Geometry: final body of the model. Coordinates: model frame, mm. Face numbers are marked on the shaded views. A direction names the side the tool comes from. Give positions to 0.01 mm unless a question says otherwise; leave off trailing zeros. Loops run counter-clockwise (first coordinate to the right, second up) from the corner with the lowest first, then second, coordinate; pieces in that order, holes last.
from build123d import *

# Parameters (mm, degrees)
PROFILESKETCH3_R               = 2.5
PROFILESKETCH3_R_2             = 2.3
PROFILEBOSS_EXTRUDE1_DEPTH     = 5.5
FILLET1_R                      = 1.5
SKETCH1_W                      = 20
SKETCH1_H                      = 15.75
SLIDINGMOUNTCUT_EXTRUDE1_DEPTH = 1


with BuildPart() as part:
    # ProfileSketch3 → ProfileBoss-Extrude1 (new body)
    with BuildSketch(Plane.XY):
        Polygon((0, 46.85), (15, 46.85), (15, 64.85), (0, 64.85), (0, 76.85), (20, 76.85), (20, 0), (0, 0), align=None)
        with Locations((7.5, 40.35)):
            Circle(PROFILESKETCH3_R, mode=Mode.SUBTRACT)
        with Locations((7.5, 71.35)):
            Circle(PROFILESKETCH3_R, mode=Mode.SUBTRACT)
        with Locations((15, 9.375)):
            Circle(PROFILESKETCH3_R_2, mode=Mode.SUBTRACT)
    extrude(amount=PROFILEBOSS_EXTRUDE1_DEPTH)

    # Fillet1
    fillet1_edges = [part.edges().sort_by_distance(p)[0] for p in [
        (7.5, 46.85, 0),
        (7.5, 64.85, 0),
    ]]
    fillet(fillet1_edges, radius=FILLET1_R)

    # Sketch1 → SlidingMountCut-Extrude1 (cut)
    with BuildSketch(Plane.XY.offset(5.5)):
        with Locations((10, 9.375)):
            Rectangle(SKETCH1_W, SKETCH1_H)
    extrude(amount=-SLIDINGMOUNTCUT_EXTRUDE1_DEPTH, mode=Mode.SUBTRACT)


solid = part.part
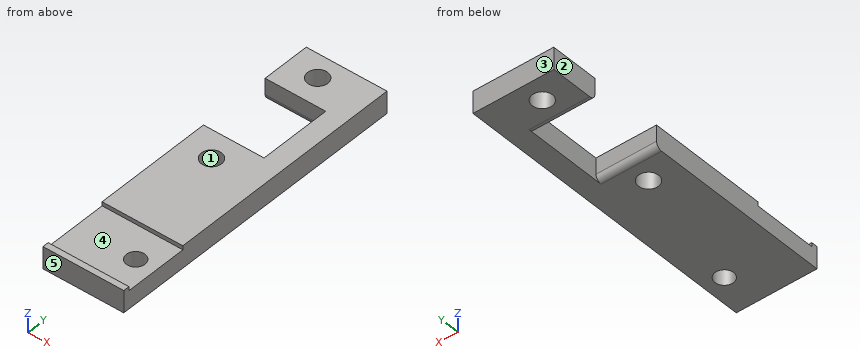
Item 1: Section query B-B on y = 40.35. Return loops of the section in (x, z).
Values follow:
outline: (0, 0) - (5, 0) - (5, 5.5) - (0, 5.5) - close; (10, 0) - (20, 0) - (20, 5.5) - (10, 5.5) - close
Item 2: Section query C-C on x = 11. Return loops of the section in (y, z).
Values follow:
outline: (0, 0) - (45.35, 0) arc R1.5 ccw to (46.85, 1.5) - (46.85, 5.5) - (17.25, 5.5) - (17.25, 4.5) - (1.5, 4.5) - (1.5, 5.5) - (0, 5.5) - close; (64.85, 1.5) arc R1.5 ccw to (66.35, 0) - (76.85, 0) - (76.85, 5.5) - (64.85, 5.5) - close
Item 3: Draft query along Y for the marked faces 1, 2 and 3. Return one class per face: +Y half, -Y half, draft (parallel to the pull), parting line (faces both ways), or undercut.
Values follow:
face 1: undercut
face 2: draft
face 3: +Y half
Item 4: Set-up query: the marked faces 4 and 5. Return all of +Z, -Z, +X, -X, +Y, -Y with unobstructed straight access to the full face (end or side cutting, diameter ignored); none if empty.
Values follow:
face 4: +Z, +X, -X
face 5: +Z, -Z, +X, -X, -Y
Item 5: Ray query, probe 1 along Y at (x, z) = (7.5, 2.9); probe 2 along Y at (x, z) = (7.5, 1.3); probe 3 along X at (y, z) = (40.5, 2.5). Return the intervals inside material, ascending.
Values follow:
probe 1: y = 0 to 37.85, 42.85 to 46.85, 64.85 to 68.85, 73.85 to 76.85
probe 2: y = 0 to 37.85, 42.85 to 46.84, 64.86 to 68.85, 73.85 to 76.85
probe 3: x = 0 to 5, 10 to 20
Item 6: Pin query (flat end, axial travel): pin 1 (1.5 mm diameter, centred on x = 2.5, y = 12.5, fed in from -Z); pin 2 (1.6 mm diameter, centred on y = 55.5, z = 2.5, fed in from -X). Return the tip coordinate at first contact, or that it passes through.
Values follow:
pin 1: stops at z = 0
pin 2: stops at x = 15
Item 7: Section query D-D on z = 2.2. Return loops of the section in (x, y) (3 decimals).
Values follow:
outline: (0, 0) - (20, 0) - (20, 76.85) - (0, 76.85) - (0, 64.85) - (15, 64.85) - (15, 46.85) - (0, 46.85) - close; hole circle Ø5 at (7.5, 40.35); hole circle Ø5 at (7.5, 71.35); hole circle Ø4.6 at (15, 9.375)
Item 8: Section query A-A on x = 7.5. Return loops of the section in (y, z).
Values follow:
outline: (0, 0) - (37.85, 0) - (37.85, 5.5) - (17.25, 5.5) - (17.25, 4.5) - (1.5, 4.5) - (1.5, 5.5) - (0, 5.5) - close; (42.85, 0) - (45.35, 0) arc R1.5 ccw to (46.85, 1.5) - (46.85, 5.5) - (42.85, 5.5) - close; (64.85, 1.5) arc R1.5 ccw to (66.35, 0) - (68.85, 0) - (68.85, 5.5) - (64.85, 5.5) - close; (73.85, 0) - (76.85, 0) - (76.85, 5.5) - (73.85, 5.5) - close
